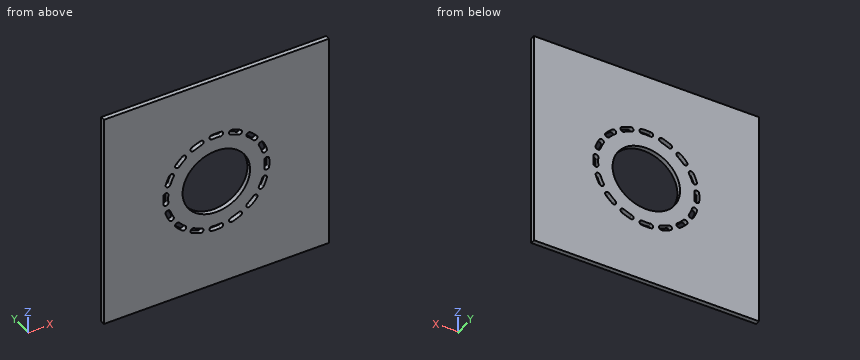
```python
from build123d import *

# Parameters (mm, degrees)
SKETCH_1_W      = 100
SKETCH_1_H      = 100
SKETCH_1_R      = 15
EXTRUDE_1_DEPTH = 2


with BuildPart() as part:
    # 草图1 → 凸台-拉伸1 (new body)
    with BuildSketch(Plane(origin=(0, 0, 0), x_dir=(1, 0, 0), z_dir=(0, 1, 0))):
        Rectangle(SKETCH_1_W, SKETCH_1_H)
        with Locations(Location((0, 0, 0), (0, 0, 270))):
            Circle(SKETCH_1_R, mode=Mode.SUBTRACT)
        with BuildLine():
            ThreePointArc((16.393351083, 13.755654847), (15.132085117, 15.132085117), (13.755654847, 16.393351083))
            ThreePointArc((13.755654847, 16.393351083), (13.620072331, 17.943066341), (15.169787589, 18.078648858))
            ThreePointArc((15.169787589, 18.078648858), (16.687720036, 16.687720036), (18.078648858, 15.169787589))
            ThreePointArc((18.078648858, 15.169787589), (17.943066341, 13.620072331), (16.393351083, 13.755654847))
        make_face(mode=Mode.SUBTRACT)
        with BuildLine():
            ThreePointArc((20.933455663, 10.897267272), (19.449820272, 11.365055714), (18.98203183, 9.881420323))
            ThreePointArc((18.98203183, 9.881420323), (19.771021996, 8.189425453), (20.409542746, 6.435104109))
            ThreePointArc((20.409542746, 6.435104109), (21.789407771, 5.716791843), (22.507720038, 7.096656868))
            ThreePointArc((22.507720038, 7.096656868), (21.803556967, 9.031329004), (20.933455663, 10.897267272))
        make_face(mode=Mode.SUBTRACT)
        with BuildLine():
            ThreePointArc((23.510194875, 2.056875529), (22.31850939, 3.05681838), (21.318566539, 1.865132895))
            ThreePointArc((21.318566539, 1.865132895), (21.4, 0), (21.318566539, -1.865132895))
            ThreePointArc((21.318566539, -1.865132895), (22.31850939, -3.05681838), (23.510194875, -2.056875529))
            ThreePointArc((23.510194875, -2.056875529), (23.6, 0), (23.510194875, 2.056875529))
        make_face(mode=Mode.SUBTRACT)
        with BuildLine():
            ThreePointArc((22.507720038, -7.096656868), (21.789407771, -5.716791843), (20.409542746, -6.435104109))
            ThreePointArc((20.409542746, -6.435104109), (19.771021996, -8.189425453), (18.98203183, -9.881420323))
            ThreePointArc((18.98203183, -9.881420323), (19.449820272, -11.365055714), (20.933455663, -10.897267272))
            ThreePointArc((20.933455663, -10.897267272), (21.803556967, -9.031329004), (22.507720038, -7.096656868))
        make_face(mode=Mode.SUBTRACT)
        with BuildLine():
            ThreePointArc((18.078648858, -15.169787589), (17.943066341, -13.620072331), (16.393351083, -13.755654847))
            ThreePointArc((16.393351083, -13.755654847), (15.132085117, -15.132085117), (13.755654847, -16.393351083))
            ThreePointArc((13.755654847, -16.393351083), (13.620072331, -17.943066341), (15.169787589, -18.078648858))
            ThreePointArc((15.169787589, -18.078648858), (16.687720036, -16.687720036), (18.078648858, -15.169787589))
        make_face(mode=Mode.SUBTRACT)
        with BuildLine():
            ThreePointArc((10.897267272, -20.933455663), (11.365055714, -19.449820272), (9.881420323, -18.98203183))
            ThreePointArc((9.881420323, -18.98203183), (8.189425453, -19.771021996), (6.435104109, -20.409542746))
            ThreePointArc((6.435104109, -20.409542746), (5.716791843, -21.789407771), (7.096656868, -22.507720038))
            ThreePointArc((7.096656868, -22.507720038), (9.031329004, -21.803556967), (10.897267272, -20.933455663))
        make_face(mode=Mode.SUBTRACT)
        with BuildLine():
            ThreePointArc((2.056875529, -23.510194875), (3.05681838, -22.31850939), (1.865132895, -21.318566539))
            ThreePointArc((1.865132895, -21.318566539), (0, -21.4), (-1.865132895, -21.318566539))
            ThreePointArc((-1.865132895, -21.318566539), (-3.05681838, -22.31850939), (-2.056875529, -23.510194875))
            ThreePointArc((-2.056875529, -23.510194875), (0, -23.6), (2.056875529, -23.510194875))
        make_face(mode=Mode.SUBTRACT)
        with BuildLine():
            ThreePointArc((-7.096656868, -22.507720038), (-5.716791843, -21.789407771), (-6.435104109, -20.409542746))
            ThreePointArc((-6.435104109, -20.409542746), (-8.189425453, -19.771021996), (-9.881420323, -18.98203183))
            ThreePointArc((-9.881420323, -18.98203183), (-11.365055714, -19.449820272), (-10.897267272, -20.933455663))
            ThreePointArc((-10.897267272, -20.933455663), (-9.031329004, -21.803556967), (-7.096656868, -22.507720038))
        make_face(mode=Mode.SUBTRACT)
        with BuildLine():
            ThreePointArc((-15.169787589, -18.078648858), (-13.620072331, -17.943066341), (-13.755654847, -16.393351083))
            ThreePointArc((-13.755654847, -16.393351083), (-15.132085117, -15.132085117), (-16.393351083, -13.755654847))
            ThreePointArc((-16.393351083, -13.755654847), (-17.943066341, -13.620072331), (-18.078648858, -15.169787589))
            ThreePointArc((-18.078648858, -15.169787589), (-16.687720036, -16.687720036), (-15.169787589, -18.078648858))
        make_face(mode=Mode.SUBTRACT)
        with BuildLine():
            ThreePointArc((-20.933455663, -10.897267272), (-19.449820272, -11.365055714), (-18.98203183, -9.881420323))
            ThreePointArc((-18.98203183, -9.881420323), (-19.771021996, -8.189425453), (-20.409542746, -6.435104109))
            ThreePointArc((-20.409542746, -6.435104109), (-21.789407771, -5.716791843), (-22.507720038, -7.096656868))
            ThreePointArc((-22.507720038, -7.096656868), (-21.803556967, -9.031329004), (-20.933455663, -10.897267272))
        make_face(mode=Mode.SUBTRACT)
        with BuildLine():
            ThreePointArc((-23.510194875, -2.056875529), (-22.31850939, -3.05681838), (-21.318566539, -1.865132895))
            ThreePointArc((-21.318566539, -1.865132895), (-21.4, 0), (-21.318566539, 1.865132895))
            ThreePointArc((-21.318566539, 1.865132895), (-22.31850939, 3.05681838), (-23.510194875, 2.056875529))
            ThreePointArc((-23.510194875, 2.056875529), (-23.6, 0), (-23.510194875, -2.056875529))
        make_face(mode=Mode.SUBTRACT)
        with BuildLine():
            ThreePointArc((-22.507720038, 7.096656868), (-21.789407771, 5.716791843), (-20.409542746, 6.435104109))
            ThreePointArc((-20.409542746, 6.435104109), (-19.771021996, 8.189425453), (-18.98203183, 9.881420323))
            ThreePointArc((-18.98203183, 9.881420323), (-19.449820272, 11.365055714), (-20.933455663, 10.897267272))
            ThreePointArc((-20.933455663, 10.897267272), (-21.803556967, 9.031329004), (-22.507720038, 7.096656868))
        make_face(mode=Mode.SUBTRACT)
        with BuildLine():
            ThreePointArc((-18.078648858, 15.169787589), (-17.943066341, 13.620072331), (-16.393351083, 13.755654847))
            ThreePointArc((-16.393351083, 13.755654847), (-15.132085117, 15.132085117), (-13.755654847, 16.393351083))
            ThreePointArc((-13.755654847, 16.393351083), (-13.620072331, 17.943066341), (-15.169787589, 18.078648858))
            ThreePointArc((-15.169787589, 18.078648858), (-16.687720036, 16.687720036), (-18.078648858, 15.169787589))
        make_face(mode=Mode.SUBTRACT)
        with BuildLine():
            ThreePointArc((-10.897267272, 20.933455663), (-11.365055714, 19.449820272), (-9.881420323, 18.98203183))
            ThreePointArc((-9.881420323, 18.98203183), (-8.189425453, 19.771021996), (-6.435104109, 20.409542746))
            ThreePointArc((-6.435104109, 20.409542746), (-5.716791843, 21.789407771), (-7.096656868, 22.507720038))
            ThreePointArc((-7.096656868, 22.507720038), (-9.031329004, 21.803556967), (-10.897267272, 20.933455663))
        make_face(mode=Mode.SUBTRACT)
        with BuildLine():
            ThreePointArc((-2.056875529, 23.510194875), (-3.05681838, 22.31850939), (-1.865132895, 21.318566539))
            ThreePointArc((-1.865132895, 21.318566539), (0, 21.4), (1.865132895, 21.318566539))
            ThreePointArc((1.865132895, 21.318566539), (3.05681838, 22.31850939), (2.056875529, 23.510194875))
            ThreePointArc((2.056875529, 23.510194875), (0, 23.6), (-2.056875529, 23.510194875))
        make_face(mode=Mode.SUBTRACT)
        with BuildLine():
            ThreePointArc((7.096656868, 22.507720038), (5.716791843, 21.789407771), (6.435104109, 20.409542746))
            ThreePointArc((6.435104109, 20.409542746), (8.189425453, 19.771021996), (9.881420323, 18.98203183))
            ThreePointArc((9.881420323, 18.98203183), (11.365055714, 19.449820272), (10.897267272, 20.933455663))
            ThreePointArc((10.897267272, 20.933455663), (9.031329004, 21.803556967), (7.096656868, 22.507720038))
        make_face(mode=Mode.SUBTRACT)
    extrude(amount=EXTRUDE_1_DEPTH)


solid = part.part
```
Design review of the part built by this model. Coordinates are the model's own, in mm. Give positions to 0.01 mm unless a question says otherwise; leave off trailing zeros. Order: outer loops, then holes, each group sorted by start corner. A loop starts at its lowest first (then second) coordinate and runs counter-clockwise, first axis right, second up. Notation, with made-up numbers: (-23, 76.5) -> (33, 76.5) arc R14 ccw to (33, 89.5) -> close; hole circle Ø5 at (18.25, 0). An arc over 180 degrees is marked (long way). Write item = value, one per line. Start each with the question number.
(1) We need section C-C on y = 0.85. State how many separate pieces and enclosed holes the cut face has, plus the area to 3 significant figures.
(2) We need section A-A on z = 0. Write out the cut boundary in (x, y).
(3) To check wall thickness, follow line 1 along X through (y, z) = (1.2, 0); line 2 along Z through (x, y) = (19, 1.5); line 3 along Z through (x, y) = (17.5, 0.85). State the ranges of each line that lie inside material, in increasing order.
(4) We need section B-B on x = 0. Write out the cut boundary in (y, z).
Numbers:
q1.separate_pieces = 1
q1.enclosed_holes = 17
q1.area = 9,090 mm^2
q2.outline = (-50, 0) -> (-23.6, 0) -> (-23.6, 2) -> (-50, 2) -> close; (-21.4, 0) -> (-15, 0) -> (-15, 2) -> (-21.4, 2) -> close; (15, 0) -> (21.4, 0) -> (21.4, 2) -> (15, 2) -> close; (23.6, 0) -> (50, 0) -> (50, 2) -> (23.6, 2) -> close
q3.line_1 = -50 to -23.6, -21.4 to -15, 15 to 21.4, 23.6 to 50
q3.line_2 = -50 to -10.93, -9.85 to 9.85, 10.93 to 50
q3.line_3 = -50 to -15.83, -13.39 to 13.39, 15.83 to 50
q4.outline = (0, -50) -> (2, -50) -> (2, -23.6) -> (0, -23.6) -> close; (0, -21.4) -> (2, -21.4) -> (2, -15) -> (0, -15) -> close; (0, 15) -> (2, 15) -> (2, 21.4) -> (0, 21.4) -> close; (0, 23.6) -> (2, 23.6) -> (2, 50) -> (0, 50) -> close
